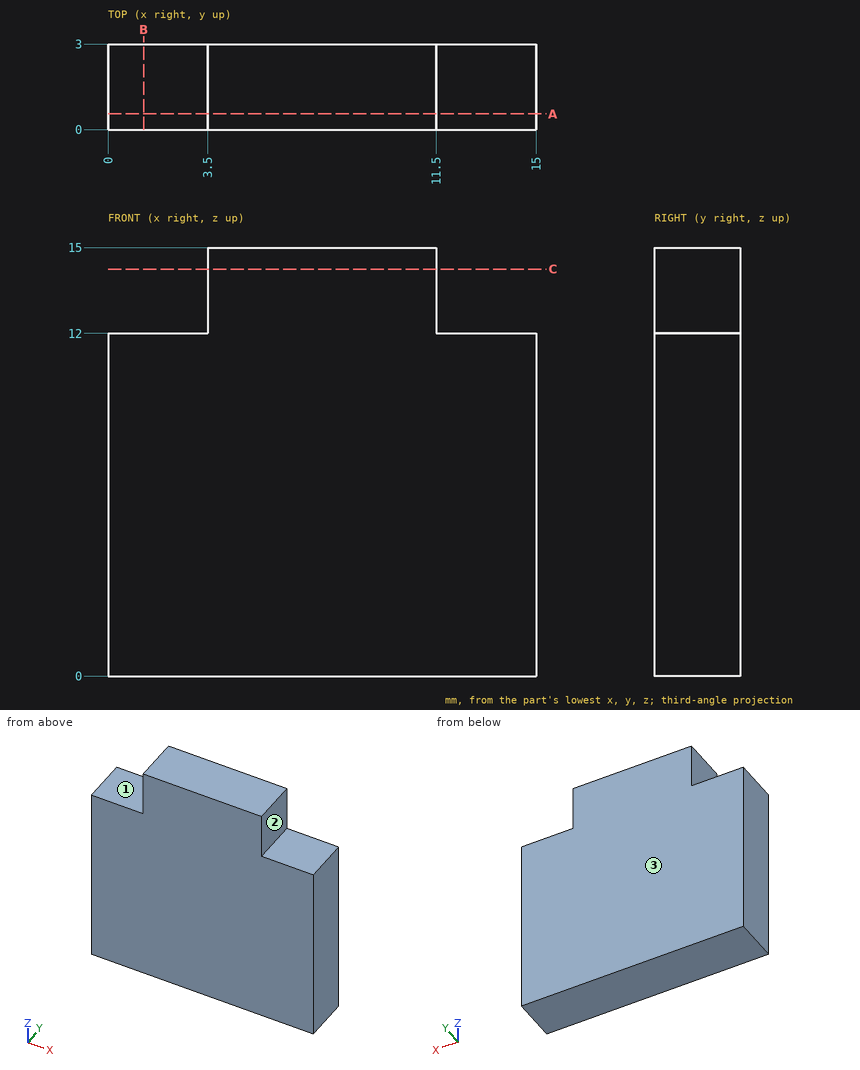
Geometry check sheet. Reference: drawing and pictorial views, mm from the part's lowest x, y, z. A direction names the side the tool comes from. Coordinates: 2 decimals unless noted, no trailing zeros. Write each loop counter-clockwise with the first axis right and the second up, starting at its lowest first coordinate (ties: lowest second). Pieces come first, ordered by that corner, then holes. Notation, with made-up numbers: (-30.5, 43.5) - (-12.5, 43.5) arc R23 cw to (-12.5, 62.5) - close; hole circle Ø11 at (86.25, 23). An arc over 180 degrees is marked (long way). Write item = value, one per line.
Q1. Cross-section at B-B (x = 1.25). Enter the section's corners in (y, z).
Answer:
outline = (0, 0) - (3, 0) - (3, 12) - (0, 12) - close
Q2. Go/stop test with a flat-tipped pin: pin 1 Ø0.9 at (y, z) = (1, 13) entering from -X. Record where the tip stops, or that it passes through.
Answer:
pin_1 = 3.5
Q3. Cross-section at A-A (y = 0.55). Enter the section's corners in (x, z).
Answer:
outline = (0, 0) - (15, 0) - (15, 12) - (11.5, 12) - (11.5, 15) - (3.5, 15) - (3.5, 12) - (0, 12) - close
Q4. Access from +Z, -Z, +X, -X, +Y, -Y to the whole of each face (thin tool, end or side, straight path). Record for the marked faces 1, 2 and 3.
Answer:
face_1 = +Z, -X, +Y, -Y
face_2 = +Z, +X, +Y, -Y
face_3 = +Z, -Z, +X, -X, +Y
Q5. Material ranges on L1, parallel to X at y = 2.95, z = 12.5; L2, parallel to Z at x = 1, y = 1, recorded low to high. Write a range as from..to.
Answer:
L1 = 3.5..11.5
L2 = 0..12
Q6. Cross-section at C-C (z = 14.25). Enter the section's corners in (x, y), plus the area to 3 significant figures.
Answer:
outline = (3.5, 0) - (11.5, 0) - (11.5, 3) - (3.5, 3) - close
area = 24.0 mm²
